Design review of the part shown in the three views and the two pictorial views. Dimensions are in mm from the part's minimum x, y and z. A direction names the side the tool comes from. Coordinates: 2 decimals unless noted, no trailing zeros. Write each loop counter-clockwise with the first axis right and the second up, starting at its lowest first coordinate (ties: lowest second). Pieces come first, ordered by that corner, then holes. Notation, with made-up numbers: M 68,59 L 73,59 A21 ccw 73,88 Z; hole C -38,78.25 d6. An arc over 180 degrees is marked long. One line per question, with ' | ' between items.
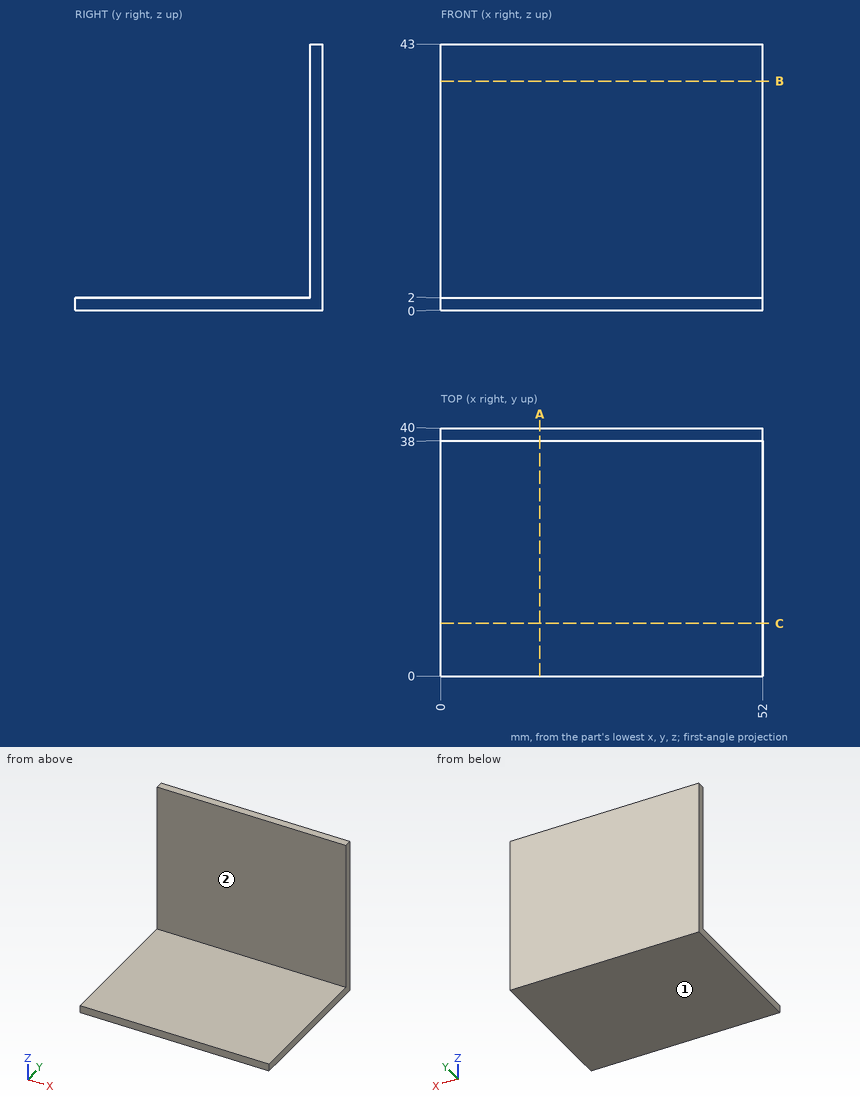
1. Machinability: for the marked faces 1 and 2, which of the approach directions +Z, -Z, +X, -X, +Y, -Y give a long, thin tool a straight path to every point of the face, cutting with its end or side? Answer none if there is none.
Computed values:
face 1: -Z, +X, -X, +Y, -Y | face 2: +Z, +X, -X, -Y
2. For line 1 along Z through (x, y) = (35, 11.5); line 2 along Y through (x, z) = (37, 26), list the stretches that pass through material, from the lowest coordinate up.
Computed values:
line 1: z = 0 to 2 | line 2: y = 38 to 40
3. Take a section at B-B on z = 37. State the section outline as (x, y) points.
Computed values:
outline: M 0,38 L 52,38 L 52,40 L 0,40 Z
4. Take a section at A-A on x = 16. State the section outline as (y, z) points.
Computed values:
outline: M 0,0 L 40,0 L 40,43 L 38,43 L 38,2 L 0,2 Z
5. Clearance check with flat-ended pins moving along their axes: P1, Ø19, axis at x = 35, y = 25.5, coming from the +Z side; P2, Ø1, axis at x = 41, z = 9.5, coming from the -Y side. State where each tip first meets the part, or that it passes through.
Computed values:
P1: stops at z = 2 | P2: stops at y = 38
6. Take a section at C-C on y = 8.5. State the section outline as (x, z) points, plus the area to 3 significant figures.
Computed values:
outline: M 0,0 L 52,0 L 52,2 L 0,2 Z | area: 104 mm2
